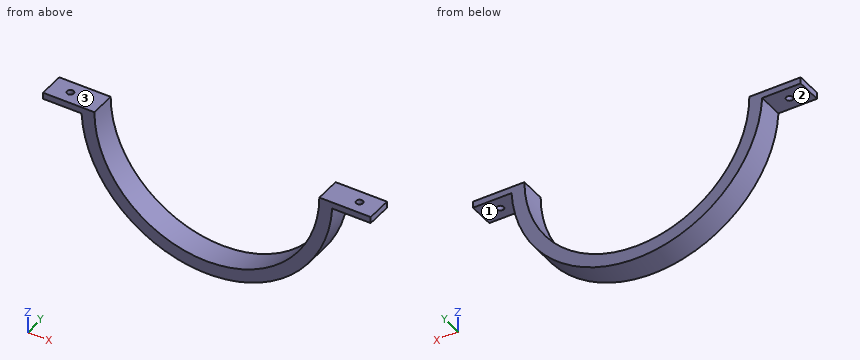
```python
from build123d import *

# Parameters (mm, degrees)
BOSS_EXTRUDE1_DEPTH = 12.7
SKETCH5_R           = 1.651
CUT_EXTRUDE1_DEPTH  = 4.175


with BuildPart() as part:
    # Sketch1 → Boss-Extrude1 (new body)
    with BuildSketch(Plane(origin=(0, 0, 0), x_dir=(1, 0, 0), z_dir=(0, 1, 0))):
        with BuildLine():
            Line((-55.5625, 0), (-80.9625, 0))
            Line((-80.9625, 0), (-80.9625, 3.175))
            Line((-80.9625, 3.175), (-61.9125, 3.175))
            ThreePointArc((-61.9125, 3.175), (0, 61.993856803), (61.9125, 3.175))
            Line((61.9125, 3.175), (80.9625, 3.175))
            Line((80.9625, 3.175), (80.9625, 0))
            Line((80.9625, 0), (55.5625, 0))
            ThreePointArc((55.5625, 0), (0, 55.5625), (-55.5625, 0))
        make_face()
    extrude(amount=BOSS_EXTRUDE1_DEPTH)

    # Sketch5 → Cut-Extrude1 (cut, through all)
    with BuildSketch(Plane(origin=(0, 0, -3.175), x_dir=(-1, 0, 0), z_dir=(0, 0, -1))):
        with Locations((71.4375, 6.35)):
            Circle(SKETCH5_R)
    cut_extrude1 = extrude(amount=-CUT_EXTRUDE1_DEPTH, mode=Mode.SUBTRACT)

    # Mirror1: Cut-Extrude1 across plane
    add(cut_extrude1.mirror(Plane(origin=(0, 0, 0), x_dir=(0, 0, 1), z_dir=(1, 0, 0))), mode=Mode.SUBTRACT)


solid = part.part
```
The model under review builds one solid part; all positions refer to its coordinate system, in mm. Face numbers are marked on the shaded views. A direction names the side the tool comes from. Round coordinates to 2 decimals unless told otherwise and drop trailing zeros. Order: outer loops, then holes, each group sorted by start corner. A loop starts at its lowest first (then second) coordinate and runs counter-clockwise, first axis right, second up.
(1) Tool access review of the marked faces 1, 2 and 3: name each direction out of +Z, -Z, +X, -X, +Y, -Y from which nothing blocks a thin tool from reaching the whole face with its end or side.
Working result:
face 1: -Z, +X, +Y, -Y
face 2: -Z, -X, +Y, -Y
face 3: +Z, +X, -X, +Y, -Y
(2) Take a section at D-D, the plane x = 0. State the section outline as (y, z) points.
Working result:
outline: (0, -61.99) - (12.7, -61.99) - (12.7, -55.56) - (0, -55.56) - close
(3) Take a section at C-C, the plane z = -41. State the section outline as (x, y) points.
Working result:
outline: (-46.5, 0) - (-37.5, 0) - (-37.5, 12.7) - (-46.5, 12.7) - close; (37.5, 0) - (46.5, 0) - (46.5, 12.7) - (37.5, 12.7) - close
(4) Wall thickness on L1, parallel to X at y = 8.75, z = -21.5; L2, parallel to Z at x = 72.5, y = 10.75 (3 decimals); L3, parallel to X at y = 6.25, z = -28: over which ranges is each line inside the solid? List them lowest first.
Working result:
L1: x = -58.15 to -51.23, 51.23 to 58.15
L2: z = -3.175 to 0
L3: x = -55.31 to -47.99, 47.99 to 55.31
(5) Take a section at A-A, the plane y = 6.35. State the section outline as (x, z) points (1 decimal), plus the area to 3 significant figures.
Working result:
outline: (-81, -3.2) - (-73.1, -3.2) - (-73.1, 0) - (-81, 0) - close; (-69.8, -3.2) - (-61.9, -3.2) arc R62 ccw to (61.9, -3.2) - (69.8, -3.2) - (69.8, 0) - (55.6, 0) arc R55.6 cw to (-55.6, 0) - (-69.8, 0) - close; (73.1, -3.2) - (81, -3.2) - (81, 0) - (73.1, 0) - close
area: 1,290 mm2
(6) For P1, Ø1.5, axis at y = 4, z = -37.5, coming from the -X side; P2, Ø1.5, axis at y = 6, z = -15, coming from the +X side; P3, Ø3, axis at x = -36.5, y = 10.5, coming from the -Z side, all flat-tipped, find the tip position at first contact; note any pin that passes through.
Working result:
P1: stops at x = -49.93
P2: stops at x = 60.33
P3: stops at z = -51.17
(7) Take a section at B-B, the plane z = -5. State the section outline as (x, y) points, plus the area to 3 significant figures.
Working result:
outline: (-61.79, 0) - (-55.34, 0) - (-55.34, 12.7) - (-61.79, 12.7) - close; (55.34, 0) - (61.79, 0) - (61.79, 12.7) - (55.34, 12.7) - close
area: 164 mm2
